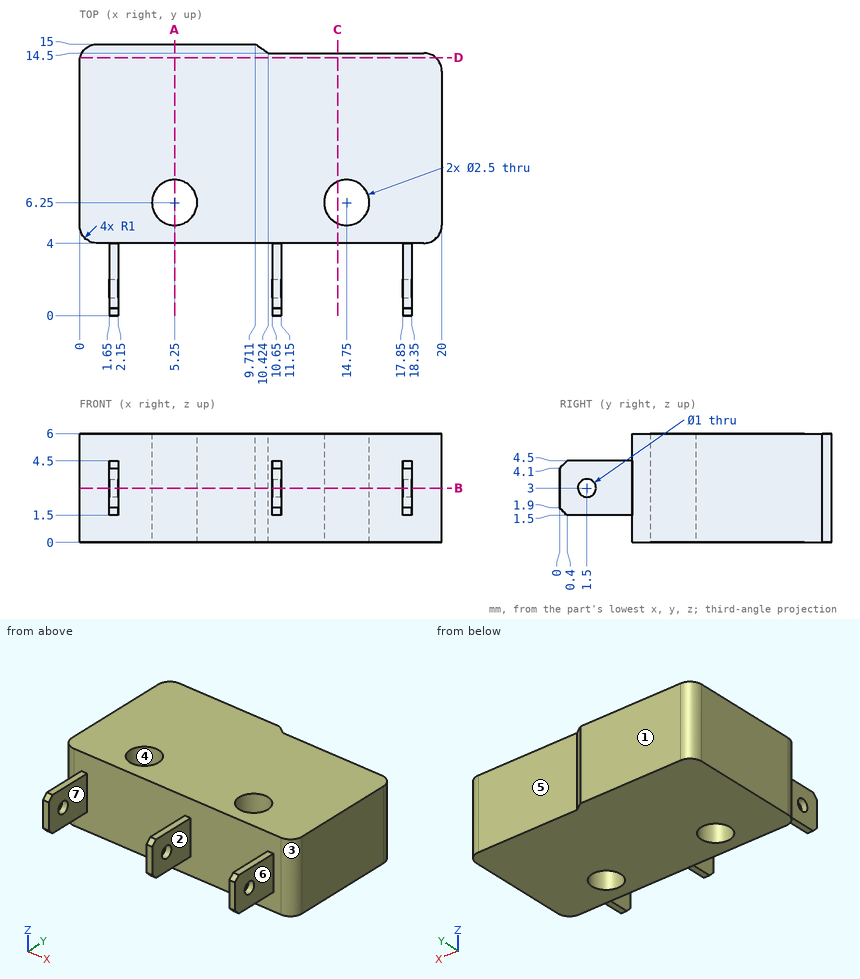
Design review of the part shown in the three views and the two pictorial views. Dimensions are in mm from the part's minimum x, y and z. A direction names the side the tool comes from. Give positions to 0.01 mm unless a question says otherwise; leave off trailing zeros. Write each loop counter-clockwise with the first axis right and the second up, starting at its lowest first coordinate (ties: lowest second). Pieces come first, ordered by that corner, then holes.
(1) Add section B-B (z = 3). Give the number of separate pieces and of enclosed holes in the cut face, and give its area (3 significant figures).
Checked values:
separate pieces: 4
enclosed holes: 2
area: 209 mm2
(2) Add section D-D (y = 14.25). Give the boundary of the cut face in (x, z).
Checked values:
outline: (0.03, 0) - (19.66, 0) - (19.66, 6) - (0.03, 6) - close
(3) Tool access review of the marked faces 5, 6 and 7: name each direction out of +Z, -Z, +X, -X, +Y, -Y from which nothing blocks a thin tool from reaching the whole face with its end or side.
Checked values:
face 5: +Z, -Z, +X, +Y
face 6: +Z, -Z, +X, -Y
face 7: +Z, -Z, -Y
(4) Mouldability with a two-part tool opening along X and no side actions: class the marked faces 1, 2, 3 and 4 as +X half, -X half, draft (parallel to the pull), parting line (faces both ways), or undercut.
Checked values:
face 1: draft
face 2: undercut
face 3: +X half
face 4: undercut
(5) Add section C-C (x = 14.25). Give the boundary of the cut face in (y, z) (1 decimal).
Checked values:
outline: (4, 0) - (5.1, 0) - (5.1, 6) - (4, 6) - close; (7.4, 0) - (14.5, 0) - (14.5, 6) - (7.4, 6) - close
(6) Clearance check with flat-ended pins moving along their axes: pin 1 Ø1.5 at (y, z) = (3, 3) entering from -X; pin 2 Ø0.6 at (x, y) = (18, 3) entering from -Z; pin 3 Ø1.5 at (y, z) = (2, 3.5) entering from +X. State where each tip first meets the part, or that it passes through.
Checked values:
pin 1: stops at x = 1.65
pin 2: stops at z = 1.5
pin 3: stops at x = 18.35
(7) Wall thickness on line 1 along Y through (x, z) = (10.85, 3); line 2 along Y through (x, z) = (14.75, 3.45); line 3 along Y through (x, z) = (17.75, 0.6): over which ranges is each line inside the solid? List them lowest first.
Checked values:
line 1: y = 0 to 1, 2 to 14.5
line 2: y = 4 to 5, 7.5 to 14.5
line 3: y = 4 to 14.5
(8) Add section A-A (x = 5.25). Give the boundary of the cut face in (y, z), and give its area (3 significant figures).
Checked values:
outline: (4, 0) - (5, 0) - (5, 6) - (4, 6) - close; (7.5, 0) - (15, 0) - (15, 6) - (7.5, 6) - close
area: 51.0 mm2
